```python
from build123d import *

# Parameters (mm, degrees)
SKETCH_R                     = 3.5
PAD_DEPTH                    = 35
SKETCH002_W                  = 48
SKETCH002_H                  = 48
SKETCH002_W_2                = 32
SKETCH002_H_2                = 32
PAD001_DEPTH                 = 6
SKETCH001_R                  = 2.25
POCKET_DEPTH                 = 7
SKETCH_LINEARPATTERN_2_R     = 3.5
PAD_LINEARPATTERN_2_DEPTH    = 35
SKETCH001_LINEARPATTERN_2_R  = 2.25
POCKET_LINEARPATTERN_2_DEPTH = 7
LINEARPATTERN001_COUNT       = 2
LINEARPATTERN001_PITCH       = 40
SKETCH003_R                  = 2.25
HOLE_DEPTH                   = 35.001
FILLET_R                     = 4
FILLET001_R                  = 3


with BuildPart() as part:
    # Sketch → Pad (new body)
    with BuildSketch(Plane.XY):
        Circle(SKETCH_R)
    pad = extrude(amount=PAD_DEPTH)

    # Sketch002 → Pad001 (join)
    with BuildSketch(Plane.XY):
        with Locations((20, 20)):
            Rectangle(SKETCH002_W, SKETCH002_H)
        with Locations((20, 20)):
            Rectangle(SKETCH002_W_2, SKETCH002_H_2, mode=Mode.SUBTRACT)
    extrude(amount=PAD001_DEPTH)

    # Sketch001 → Pocket (cut)
    with BuildSketch(Plane.XY.offset(35)):
        Circle(SKETCH001_R)
    pocket = extrude(amount=-POCKET_DEPTH, mode=Mode.SUBTRACT)

    # Sketch LinearPattern 2 → Pad LinearPattern 2 (add)
    with BuildSketch(Plane(origin=(40, 0, 0), x_dir=(1, 0, 0), z_dir=(0, 0, 1))):
        Circle(SKETCH_LINEARPATTERN_2_R)
    pad_linearpattern_2 = extrude(amount=PAD_LINEARPATTERN_2_DEPTH)

    # Sketch001 LinearPattern 2 → Pocket LinearPattern 2 (cut)
    with BuildSketch(Plane(origin=(40, 0, 35), x_dir=(1, 0, 0), z_dir=(0, 0, 1))):
        Circle(SKETCH001_LINEARPATTERN_2_R)
    pocket_linearpattern_2 = extrude(amount=-POCKET_LINEARPATTERN_2_DEPTH, mode=Mode.SUBTRACT)

    # LinearPattern001: Pad, Pocket, Pad LinearPattern 2, Pocket LinearPattern 2 ×2
    with Locations(*[(0, i * LINEARPATTERN001_PITCH, 0) for i in range(1, LINEARPATTERN001_COUNT)]):
        add(pad)
        add(pocket, mode=Mode.SUBTRACT)
        add(pad_linearpattern_2)
        add(pocket_linearpattern_2, mode=Mode.SUBTRACT)

    # Sketch003 → Hole (cut, through all)
    with BuildSketch(Plane.XY):
        with Locations((10, 40)):
            Circle(SKETCH003_R)
        with Locations((30, 40)):
            Circle(SKETCH003_R)
        with Locations((30, 0)):
            Circle(SKETCH003_R)
        with Locations((10, 0)):
            Circle(SKETCH003_R)
    extrude(amount=HOLE_DEPTH, mode=Mode.SUBTRACT)

    # Fillet
    fillet_edges = [part.edges().sort_by_distance(p)[0] for p in [
        (-4, -4, 3),
        (44, -4, 3),
        (-4, 44, 3),
        (44, 44, 3),
    ]]
    fillet(fillet_edges, radius=FILLET_R)

    # Fillet001
    fillet001_edges = [part.edges().sort_by_distance(p)[0] for p in [
        (4, 36, 3),
        (36, 36, 3),
        (36, 4, 3),
        (4, 4, 3),
    ]]
    fillet(fillet001_edges, radius=FILLET001_R)


solid = part.part
```
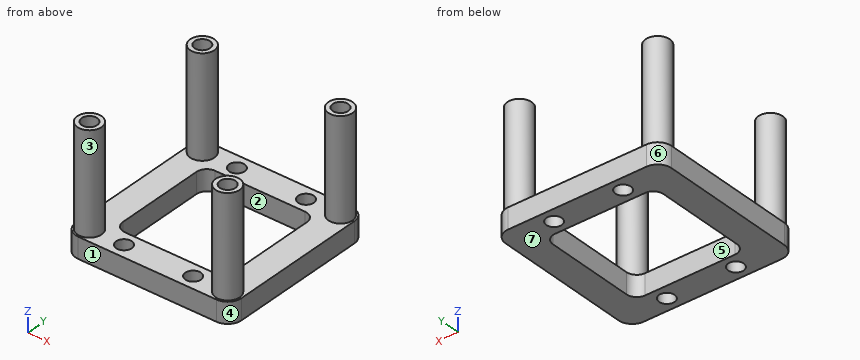
Could you check a few things on this model? Use its own coordinates, in mm. Face numbers are marked on the shaded views. A direction names the side the tool comes from. Give positions to 0.01 mm unless a question says otherwise; leave off trailing zeros. Write each loop counter-clockwise with the first axis right and the second up, starting at its lowest first coordinate (ties: lowest second). Pieces come first, ordered by that corner, then holes. Notation, with made-up numbers: (-39.75, -35.75) - (-23.75, -35.75) arc R24 ccw to (-23.75, -23.75) - close; hole circle Ø1 at (-0.75, 58.5). An arc over 180 degrees is marked (long way). One line per item, written item: value. Start each with the question number.
Item 1: Imagine slicing it at C-C, the plane x = 30. List the corners of the cut face in (y, z) for me.
Item 2: I'm going to push flat-ended pins straight in: pin 1 (2 mm diameter, centred on x = 41, y = 39.5, fed in from +Z); pin 2 (12 mm diameter, centred on y = 12, z = 13.5, fed in from +X); pin 3 (5 mm diameter, centred on x = 10, y = 0, fed in from +Z). Where does each tip first touch, or does it pass through?
Item 3: If we mould it in two halves opening along Y, with no side actions, what happens to the marked faces 4, 5, 6 and 7? For each: +Y half, -Y half, draft (parallel to the pull), parting line (faces both ways), or undercut.
Item 4: Imagine slicing it at D-D, the plane z = 15. List the corners of the cut face in (x, y) for me.
Item 5: Please list where these lines run through material, in increasing order: line 1 (Y direction, x = 10, z = 4.35); line 2 (Y direction, x = 40, z = 30); line 3 (X direction, y = 0, z = 2.95). Write a range as from..to.
Item 6: Which directions (+Z, -Z, +X, -X, +Y, -Y) give clear straight access to the entire face, cutting with the end or side of a thin tool? Please do the marked faces 1, 2 and 3.
Item 7: Imagine slicing it at A-A, the plane y = 29.5. List the corners of the cut face in (x, z) for me.
Geometry says:
1. outline: (-4, 0) - (-2.25, 0) - (-2.25, 6) - (-4, 6) - close; (2.25, 0) - (4, 0) - (4, 6) - (2.25, 6) - close; (36, 0) - (37.75, 0) - (37.75, 6) - (36, 6) - close; (42.25, 0) - (44, 0) - (44, 6) - (42.25, 6) - close
2. pin 1: z = 28
2. pin 2: through
2. pin 3: z = 6
3. face 4: -Y half
3. face 5: undercut
3. face 6: +Y half
3. face 7: draft
4. outline: circle Ø7 at (0, 0); circle Ø7 at (0, 40); circle Ø7 at (40, 0); circle Ø7 at (40, 40)
5. line 1: -4..-2.25, 2.25..4, 36..37.75, 42.25..44
5. line 2: -3.5..-2.25, 2.25..3.5, 36.5..37.75, 42.25..43.5
5. line 3: -4..7.75, 12.25..27.75, 32.25..44
6. face 1: +Z, -Z, +X, -X, -Y
6. face 2: +Z, -Z
6. face 3: +Z
7. outline: (-4, 0) - (4, 0) - (4, 6) - (-4, 6) - close; (36, 0) - (44, 0) - (44, 6) - (36, 6) - close
